Geometry: final body of the model. Coordinates: model frame, mm. Coordinates: 2 decimals unless noted, no trailing zeros. Write each loop counter-clockwise with the first axis right and the second up, starting at its lowest first coordinate (ties: lowest second). Pieces come first, ordered by that corner, then holes. Notation, with made-up numbers: (44, 32.25) - (80, 32.25) arc R15 ccw to (80, 39.25) - close; hole circle Ø2 at (-15.5, 28). An arc over 180 degrees is marked (long way). Answer as a JSON object with one key per item and string values. Group by question number.
Item 1: Section A-A on y = -29. Return loops of the section in (x, z).
Item 2: Line query: line 1 along X through (y, z) = (31, 0.85); line 2 along Y through (x, z) = (27, 0.6); line 3 along X through (y, z) = (-2.5, 1.4). Output: solid intervals per line, ascending. Write a range as from..to.
Item 3: Section B-B on y = 18.5. Return loops of the section in (x, z), and give its area (3 significant figures).
```python
from build123d import *

# Parameters (mm, degrees)
SKETCH1_R              = 5.42
BOSS_EXTRUDE1_DEPTH    = 2.03
BOSS_EXTRUDE1_2_DEPTH  = 2.03
BOSS_EXTRUDE1_3_DEPTH  = 2.03
BOSS_EXTRUDE1_4_DEPTH  = 2.03
BOSS_EXTRUDE1_5_DEPTH  = 2.03
BOSS_EXTRUDE1_6_DEPTH  = 2.03
BOSS_EXTRUDE1_7_DEPTH  = 2.03
BOSS_EXTRUDE1_8_DEPTH  = 2.03
BOSS_EXTRUDE1_9_DEPTH  = 2.03
BOSS_EXTRUDE1_10_DEPTH = 2.03
SKETCH2_R              = 34.53
SKETCH2_R_2            = 30.53
BOSS_EXTRUDE2_DEPTH    = 2.03
SKETCH3_R              = 9
BOSS_EXTRUDE3_DEPTH    = 2.03


with BuildPart() as part:
    # Sketch1 → Boss-Extrude1 (new body)
    with BuildSketch(Plane.XY):
        with Locations((0, -32.53)):
            Circle(SKETCH1_R)
    extrude(amount=BOSS_EXTRUDE1_DEPTH)



with BuildPart() as body_2:
    # Sketch1 → Boss-Extrude1 2 (new body)
    with BuildSketch(Plane.XY):
        with Locations((-19.120654257, -26.317322827)):
            Circle(SKETCH1_R)
    extrude(amount=BOSS_EXTRUDE1_2_DEPTH)


with BuildPart() as body_3:
    # Sketch1 → Boss-Extrude1 3 (new body)
    with BuildSketch(Plane.XY):
        with Locations((-30.937868475, -10.052322827)):
            Circle(SKETCH1_R)
    extrude(amount=BOSS_EXTRUDE1_3_DEPTH)


with BuildPart() as body_4:
    # Sketch1 → Boss-Extrude1 4 (new body)
    with BuildSketch(Plane.XY):
        with Locations((-30.937868475, 10.052322827)):
            Circle(SKETCH1_R)
    extrude(amount=BOSS_EXTRUDE1_4_DEPTH)


with BuildPart() as body_5:
    # Sketch1 → Boss-Extrude1 5 (new body)
    with BuildSketch(Plane.XY):
        with Locations((-19.120654257, 26.317322827)):
            Circle(SKETCH1_R)
    extrude(amount=BOSS_EXTRUDE1_5_DEPTH)


with BuildPart() as body_6:
    # Sketch1 → Boss-Extrude1 6 (new body)
    with BuildSketch(Plane.XY):
        with Locations((0, 32.53)):
            Circle(SKETCH1_R)
    extrude(amount=BOSS_EXTRUDE1_6_DEPTH)


with BuildPart() as body_7:
    # Sketch1 → Boss-Extrude1 7 (new body)
    with BuildSketch(Plane.XY):
        with Locations((19.120654257, 26.317322827)):
            Circle(SKETCH1_R)
    extrude(amount=BOSS_EXTRUDE1_7_DEPTH)


with BuildPart() as body_8:
    # Sketch1 → Boss-Extrude1 8 (new body)
    with BuildSketch(Plane.XY):
        with Locations((30.937868475, 10.052322827)):
            Circle(SKETCH1_R)
    extrude(amount=BOSS_EXTRUDE1_8_DEPTH)


with BuildPart() as body_9:
    # Sketch1 → Boss-Extrude1 9 (new body)
    with BuildSketch(Plane.XY):
        with Locations((30.937868475, -10.052322827)):
            Circle(SKETCH1_R)
    extrude(amount=BOSS_EXTRUDE1_9_DEPTH)


with BuildPart() as body_10:
    # Sketch1 → Boss-Extrude1 10 (new body)
    with BuildSketch(Plane.XY):
        with Locations((19.120654257, -26.317322827)):
            Circle(SKETCH1_R)
    extrude(amount=BOSS_EXTRUDE1_10_DEPTH)


with BuildPart() as part_1:
    add(part.part)

    add(body_2.part)  # Boss-Extrude2 merges body 2

    add(body_3.part)  # Boss-Extrude2 merges body 3

    add(body_4.part)  # Boss-Extrude2 merges body 4

    add(body_5.part)  # Boss-Extrude2 merges body 5

    add(body_6.part)  # Boss-Extrude2 merges body 6

    add(body_7.part)  # Boss-Extrude2 merges body 7

    add(body_8.part)  # Boss-Extrude2 merges body 8

    add(body_9.part)  # Boss-Extrude2 merges body 9

    add(body_10.part)  # Boss-Extrude2 merges body 10
    # Sketch2 → Boss-Extrude2 (add)
    with BuildSketch(Plane.XY.offset(2.03)):
        Circle(SKETCH2_R)
        Circle(SKETCH2_R_2, mode=Mode.SUBTRACT)
    extrude(amount=-BOSS_EXTRUDE2_DEPTH)

    # Sketch3 → Boss-Extrude3 (add)
    with BuildSketch(Plane.XY.offset(2.03)):
        with Locations((-30.937868475, -10.052322827)):
            Circle(SKETCH3_R)
    boss_extrude3 = extrude(amount=-BOSS_EXTRUDE3_DEPTH)

    # Mirror1: Boss-Extrude3 across plane
    add(boss_extrude3.mirror(Plane(origin=(0, 0, 0), x_dir=(0, 0, 1), z_dir=(1, 0, 0))))


solid = part_1.part
```
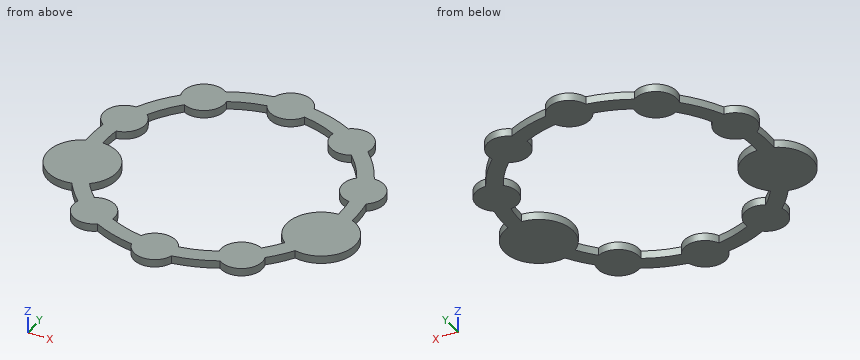
Checks:
{
 "1": {"outline": "(-23.83, 0) - (-9.54, 0) - (-9.54, 2.03) - (-23.83, 2.03) - close; (-4.11, 0) - (4.11, 0) - (4.11, 2.03) - (-4.11, 2.03) - close; (9.54, 0) - (23.83, 0) - (23.83, 2.03) - (9.54, 2.03) - close"},
 "2": {"line 1": "-21.85..-16.39, -15.21..15.21, 16.39..21.85", "line 2": "-21.52..-1.96, 6.33..13.78, 14.25..21.52", "line 3": "-35.83..-26.04, 26.04..35.83"},
 "3": {"outline": "(-29.16, 0) - (-24.29, 0) - (-24.29, 2.03) - (-29.16, 2.03) - close; (24.29, 0) - (29.16, 0) - (29.16, 2.03) - (24.29, 2.03) - close", "area": "19.8 mm^2"}
}
